Verification items for the finished model (mm, model axes). A direction names the side the tool comes from. Round coordinates to 2 decimals unless told otherwise and drop trailing zeros. Order: outer loops, then holes, each group sorted by start corner. A loop starts at its lowest first (then second) coordinate and runs counter-clockwise, first axis right, second up. Notation, with made-up numbers: M 28,-31.75 L 56,-31.75 A32 ccw 56,-5.75 Z; hole C 16.25,80.25 d3. An arc over 180 degrees is marked long. Use one line per item in the form item = value. Start each with the question number.
Item 1: Thickness scan on probe 1 along Z at (x, y) = (-36.75, 29); probe 2 along Y at (x, z) = (-38.25, -15.5); probe 3 along X at (y, z) = (32.25, -18.5). Record the ranges inside material, lowest first. Write a range as [from, to].
Item 2: Cross-section at A-A on x = -35.25. Enter the section's corners in (y, z), then the cut area to 3 significant figures.
Item 3: Cross-section at B-B on z = -41. Enter the section's corners in (x, y), then the cut area to 3 significant figures.
Item 4: Tool access check on faces 1 (the flat face through (-34.248, 31, -43)), 2 (the cylindrical face through (-37.495, 32.68, -33.965)). Record the directions out of +Z, -Z, +X, -X, +Y, -Y that give a thin tool (end or side, any length) a straight path to the whole face; none if there is none.
Item 5: Release check for a two-part mould opening along Z. For faces 3 (the flat face through (-36, 32, -25)), 4 (the flat face through (-36, 32, -28)), 5 (the flat face through (-38, 27.5, -6)) record: +Z half, -Z half, draft (parallel to the pull), parting line (faces both ways), or undercut.
Item 6: Cross-section at C-C on z = -16. Enter the section's corners in (x, y).
Autodesk Inventor part; units mm, degrees
ref_plane "Plano de trabajo1" through (0, 0, 0) normal (0, 0, 1) x (1, 0, 0)
ref_plane "Plano de trabajo2" through (-44.5, -51.5, -48) normal (0, 0, -1) x (0, 1, 0)
ref_plane "Plano de trabajo3" through (0, 0, -45.1) normal (0, 0, 1) x (1, 0, 0)
ref_plane "Plano de trabajo1" through (0, 0, 0) normal (0, 0, 1) x (1, 0, 0)
sketch "Boceto1" plane through (0, 0, 0) normal (0, 0, 1) x (1, 0, 0)
  circle A0 centre (-38.2477, 31.5) radius 1.5 construction
  circle A1 centre (-38.2477, 31.5) radius 1.4
  point P0 (0, 0)
  dimension "d2" = 0.1
ref_plane "Plano de trabajo2" through (-44.5, -51.5, -48) normal (0, 0, -1) x (0, 1, 0)
extrude "Extrusión1" add sketch "Boceto1" against normal up to surface (48 mm away)
ref_plane "Plano de trabajo3" through (0, 0, -45.1) normal (0, 0, 1) x (1, 0, 0)
sketch "Boceto2" plane through (0, 0, -45.1) normal (0, 0, 1) x (1, 0, 0)
  circle A0 centre (-38.2477, 31.5) radius 1.4 construction
  line L0 (-34.2477, 35.5) -> (-42.2477, 35.5)
  line L1 (-42.2477, 35.5) -> (-42.2477, 27.5)
  line L2 (-42.2477, 27.5) -> (-34.2477, 27.5)
  line L3 (-34.2477, 27.5) -> (-34.2477, 35.5)
  line L4 (-34.2477, 35.5) -> (-42.2477, 27.5) construction
  line L5 (-42.2477, 35.5) -> (-34.2477, 27.5) construction
  point P0 (0, 0)
  dimension "d3" = 8
  dimension "d4" = 8
extrude "Extrusión2" add sketch "Boceto2" along normal blind 5
chamfer "Chaflán1" distance 2 angle 45 4 edges at (-42.2477, 35.5, -42.6) (-34.2477, 35.5, -42.6) (-34.2477, 27.5, -42.6) (-42.2477, 27.5, -42.6)
ref_plane "Plano de trabajo4" through (0, 0, -3.1) normal (0, 0, -1) x (-1, 0, 0)
sketch "Boceto3" plane through (0, 0, -3.1) normal (0, 0, -1) x (-1, 0, 0)
  circle A0 centre (38.2477, 31.5) radius 1.4 construction
  line L0 (34.2477, 27.5) -> (42.2477, 27.5)
  line L1 (42.2477, 27.5) -> (42.2477, 35.5)
  line L2 (42.2477, 35.5) -> (34.2477, 35.5)
  line L3 (34.2477, 35.5) -> (34.2477, 27.5)
  line L4 (34.2477, 27.5) -> (42.2477, 35.5) construction
  line L5 (42.2477, 27.5) -> (34.2477, 35.5) construction
  point P0 (0, 0)
  dimension "d10" = 8
  dimension "d11" = 8
extrude "Extrusión3" add sketch "Boceto3" along normal blind 5
chamfer "Chaflán2" distance 2 angle 45 4 edges at (-42.2477, 35.5, -5.6) (-34.2477, 35.5, -5.6) (-34.2477, 27.5, -5.6) (-42.2477, 27.5, -5.6)
ref_plane "Plano de trabajo5" through (-38.2477, 31.5, -24) normal (0, 0, -1) x (-1, 0, 0)
sketch "Boceto4" plane through (-38.2477, 31.5, -24) normal (0, 0, -1) x (-1, 0, 0)
  circle A0 centre (0, 0) radius 1.5 construction
  line L0 (-4, -4) -> (4, -4)
  line L1 (4, -4) -> (4, 4)
  line L2 (4, 4) -> (-4, 4)
  line L3 (-4, 4) -> (-4, -4)
  line L4 (-4, -4) -> (4, 4) construction
  line L5 (4, -4) -> (-4, 4) construction
  point P0 (-38.2477, -31.5)
  dimension "d17" = 8
  dimension "d18" = 8
extrude "Extrusión4" add sketch "Boceto4" along normal mid plane 8
chamfer "Chaflán3" distance 2 angle 45 4 edges at (-42.2477, 35.5, -24) (-42.2477, 27.5, -24) (-34.2477, 35.5, -24) (-34.2477, 27.5, -24)
sketch "Boceto5" plane through (-38.2477, 31.5, -24) normal (0, 0, -1) x (-1, 0, 0)
  circle A0 centre (0, 0) radius 1.4 construction
  line L0 (-4, 4) -> (4, 4)
  line L1 (4, 4) -> (4, -4)
  line L2 (4, -4) -> (-4, -4)
  line L3 (-4, -4) -> (-4, 4)
  line L4 (-4, 4) -> (4, -4) construction
  line L5 (4, 4) -> (-4, -4) construction
  circle A1 centre (0, 0) radius 1.4
  point P0 (-38.2477, -31.5)
  dimension "d24" = 8
  dimension "d25" = 8
extrude "Extrusión5" cut sketch "Boceto5" along normal mid plane 2
properties part number "EjeFrontalGrúa"
Output values:
q1.probe_1 = [-45.1, -40.1], [-28, -25], [-23, -20], [-8.1, -3.1]
q1.probe_2 = [30.1, 32.9]
q1.probe_3 = [-39.43, -37.07]
q2.outline = M 28.5,-45.1 L 34.5,-45.1 L 34.5,-40.1 L 28.5,-40.1 Z; M 28.5,-28 L 34.5,-28 L 34.5,-25 L 28.5,-25 Z; M 28.5,-23 L 34.5,-23 L 34.5,-20 L 28.5,-20 Z; M 28.5,-8.1 L 34.5,-8.1 L 34.5,-3.1 L 28.5,-3.1 Z
q2.area = 96.1 mm2
q3.outline = M -42.25,29.5 L -40.25,27.5 L -36.25,27.5 L -34.25,29.5 L -34.25,33.5 L -36.25,35.5 L -40.25,35.5 L -42.25,33.5 Z
q3.area = 56.0 mm2
q4.face_1 = +Z, -Z, +X, +Y, -Y
q4.face_2 = none
q5.face_3 = undercut
q5.face_4 = undercut
q5.face_5 = draft
q6.outline = C -38.25,31.5 d2.8
